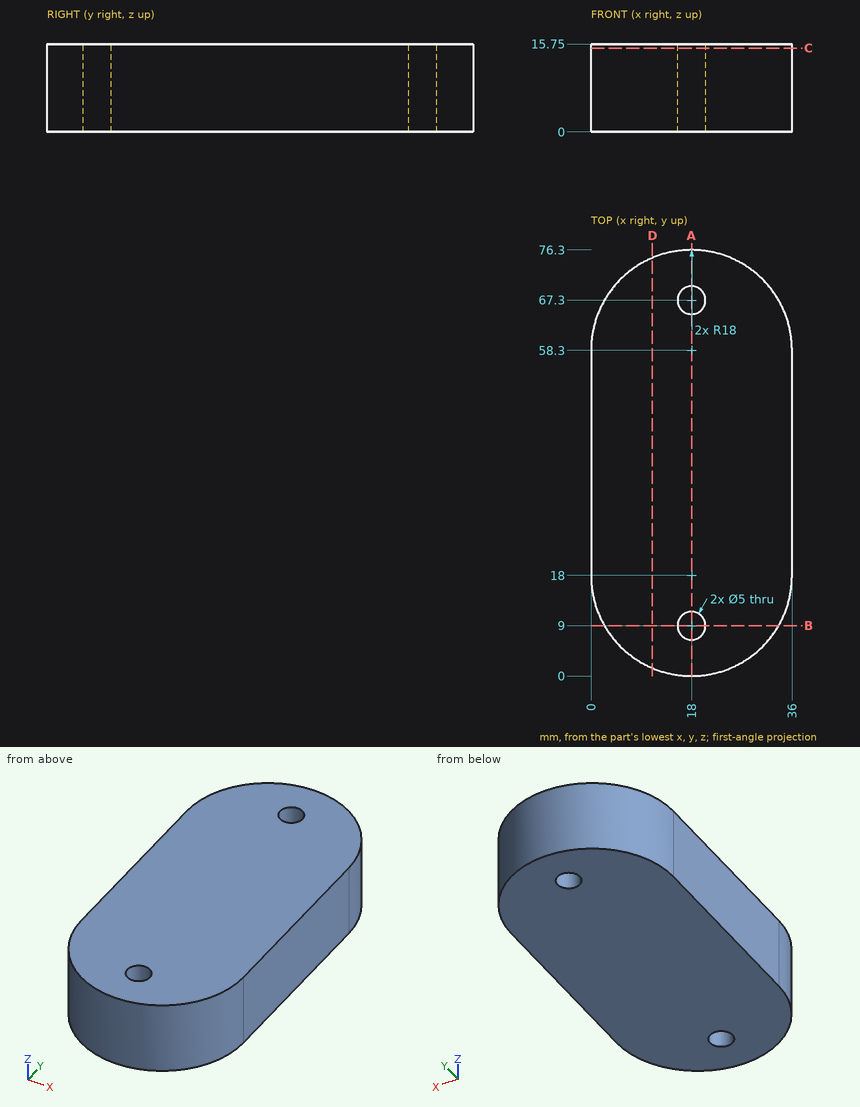
Study the drawing (mm; zero at the part's minimum x, y, z) and answer. Give positions to 0.01 mm unless a question says otherwise; leave off trailing zeros. Loops run counter-clockwise (first coordinate to the right, second up) from the corner with the lowest first, then second, coordinate; pieces in that order, holes last. Notation, with made-up numbers: M 5,70 L 56,70 A31 cw 56,96 Z; hole C 22,-39.75 d9. An arc over 180 degrees is marked long. Use CSV: the item, a comma, the result in double quotes.
1) Find section C-C on z = 15. Write down the section's boundary in (x, y), plus the area to 3 significant figures.
Answer:
outline,"M 0,18 A18 ccw 36,18 L 36,58.3 A18 ccw 0,58.3 Z; hole C 18,9 d5; hole C 18,67.3 d5"
area,"2,430 mm^2"
2) Given P1, Ø1.5, axis at x = 31, z = 5, coming from the +Y side; P2, Ø4, axis at x = 13, z = 9, coming from the +Y side; P3, Ø3, axis at x = 18, y = 67.3, coming from the +Z side; P4, Ø5, axis at y = 10, z = 6, coming from the -X side, each flat-ended and moving along its own axis, determine where each tip first touches the part or whether it passes through.
Answer:
P1,"y = 71.49"
P2,"y = 76.05"
P3,"through"
P4,"x = 0.86"
3) Find section D-D on x = 11. Write down the section's boundary in (y, z), plus the area to 3 significant figures.
Answer:
outline,"M 1.42,0 L 74.88,0 L 74.88,15.75 L 1.42,15.75 Z"
area,"1,160 mm^2"
4) Consider L1, parallel to Y at x = 18, z = 7; L2, parallel to Y at x = 16.5, z = 8.25; L3, parallel to Y at x = 2, z = 1.5. Determine where each line is inside the solid, lowest interval first.
Answer:
L1,"0 to 6.5, 11.5 to 64.8, 69.8 to 76.3"
L2,"0.06 to 7, 11 to 65.3, 69.3 to 76.24"
L3,"9.75 to 66.55"
5) Find section B-B on y = 9. Write down the section's boundary in (x, z).
Answer:
outline,"M 2.41,0 L 15.5,0 L 15.5,15.75 L 2.41,15.75 Z; M 20.5,0 L 33.59,0 L 33.59,15.75 L 20.5,15.75 Z"
6) Find section A-A on x = 18. Write down the section's boundary in (y, z), plus the area to 3 significant figures.
Answer:
outline,"M 0,0 L 6.5,0 L 6.5,15.75 L 0,15.75 Z; M 11.5,0 L 64.8,0 L 64.8,15.75 L 11.5,15.75 Z; M 69.8,0 L 76.3,0 L 76.3,15.75 L 69.8,15.75 Z"
area,"1,040 mm^2"
